```python
from build123d import *

# Parameters (mm, degrees)
F1_DEPTH  = 25
F3_DEPTH  = 75
F5_DEPTH  = 10
F7_R      = 13.8307060356
F7_R_2    = 7.44
F8_DEPTH  = 10
F9_DEPTH  = 35.001
F11_DEPTH = 20
F13_R     = 35.5
F14_DEPTH = 130
F15_R     = 20.5
F16_DEPTH = 223.001
F18_R     = 35.5
F19_DEPTH = 130
F20_R     = 20.5
F21_DEPTH = 210.001
F22_SIZE  = 2


with BuildPart() as f1:
    # F0 (on Top) → F1 (new body)
    with BuildSketch(Plane.XY):
        with BuildLine():
            Line((-190, 0), (-10, 0))
            ThreePointArc((-10, 0), (-2.9289321881, 2.9289321881), (0, 10))
            Line((0, 10), (0, 203))
            ThreePointArc((0, 203), (-2.9289321881, 210.0710678119), (-10, 213))
            Line((-10, 213), (-190, 213))
            ThreePointArc((-190, 213), (-197.0710678119, 210.0710678119), (-200, 203))
            Line((-200, 203), (-200, 10))
            ThreePointArc((-200, 10), (-197.0710678119, 2.9289321881), (-190, 0))
        make_face()
    extrude(amount=F1_DEPTH)

    # F2 (on face) → F3 (join)
    with BuildSketch(Plane.XY.offset(25)):
        with BuildLine():
            Line((0, 155.0000011921), (0, 170))
            Line((0, 170), (-80, 170))
            ThreePointArc((-80, 170), (-106.3603896932, 106.3603896932), (-170, 80))
            Line((-170, 80), (-170, 0))
            Line((-170, 0), (-155, 0))
            Line((-155, 0), (-155, 66.0769515459))
            ThreePointArc((-155, 66.0769515459), (-95.7537875496, 95.7537884012), (-66.0769513738, 155.0000011921))
            Line((-66.0769513738, 155.0000011921), (0, 155.0000011921))
        make_face()
    extrude(amount=F3_DEPTH)

    # F4 (on face) → F5 (join)
    with BuildSketch(Plane.XY.offset(25)):
        with BuildLine():
            Line((0, 60), (-45, 60))
            ThreePointArc((-45, 60), (-55.6066017178, 55.6066017178), (-60, 45))
            Line((-60, 45), (-60, 0))
            Line((-60, 0), (-10, 0))
            ThreePointArc((-10, 0), (-2.9289321881, 2.9289321881), (0, 10))
            Line((0, 10), (0, 60))
        make_face()
    extrude(amount=F5_DEPTH)

    # F7 (on face) → F8 (cut)
    with BuildSketch(Plane.XY.offset(35)):
        with Locations((-30, 30)):
            Circle(F7_R)
        with Locations((-30, 30)):
            Circle(F7_R_2, mode=Mode.SUBTRACT)
    extrude(amount=-F8_DEPTH, mode=Mode.SUBTRACT)

    # F7 (on face) → F9 (cut, through all)
    with BuildSketch(Plane.XY.offset(35)):
        with Locations((-30, 30)):
            Circle(F7_R_2)
    extrude(amount=-F9_DEPTH, mode=Mode.SUBTRACT)

    # F10 (on face) → F11 (cut)
    with BuildSketch(Plane.XY.offset(25)):
        with BuildLine():
            ThreePointArc((-78, 9), (-71.6360389693, 11.6360389693), (-69, 18))
            Line((-69, 18), (-69, 45))
            ThreePointArc((-69, 45), (-61.9705627485, 61.9705627485), (-45, 69))
            Line((-45, 69), (-18, 69))
            ThreePointArc((-18, 69), (-11.6360389693, 71.6360389693), (-9, 78))
            Line((-9, 78), (-9, 137.0000011921))
            ThreePointArc((-9, 137.0000011921), (-11.6360389693, 143.3639622228), (-18, 146.0000011921))
            Line((-18, 146.0000011921), (-51.5094937192, 146.0000011921))
            ThreePointArc((-51.5094937192, 146.0000011921), (-56.9532191654, 144.1669986991), (-60.1795307641, 139.4146352512))
            ThreePointArc((-60.1795307641, 139.4146352512), (-89.3898265392, 89.3898273502), (-139.4146341463, 60.1795310719))
            ThreePointArc((-139.4146341463, 60.1795310719), (-144.1669975344, 56.9532194614), (-146, 51.5094940512))
            Line((-146, 51.5094940512), (-146, 18))
            ThreePointArc((-146, 18), (-143.3639610307, 11.6360389693), (-137, 9))
            Line((-137, 9), (-78, 9))
        make_face()
    extrude(amount=-F11_DEPTH, mode=Mode.SUBTRACT)

    # F13 (on offset) → F14 (join)
    with BuildSketch(Plane.XZ.offset(10)):
        with Locations((-162.5, 100)):
            Circle(F13_R)
    extrude(amount=-F14_DEPTH)

    # F15 (on face) → F16 (cut, through all)
    with BuildSketch(Plane.XZ.offset(10)):
        with Locations((-162.5, 100)):
            Circle(F15_R)
    extrude(amount=-F16_DEPTH, mode=Mode.SUBTRACT)

    # F18 (on offset) → F19 (join)
    with BuildSketch(Plane.YZ.offset(10)):
        with Locations((162.5, 100)):
            Circle(F18_R)
    extrude(amount=-F19_DEPTH)

    # F20 (on face) → F21 (cut, through all)
    with BuildSketch(Plane.YZ.offset(10)):
        with Locations((162.5, 100)):
            Circle(F20_R)
    extrude(amount=-F21_DEPTH, mode=Mode.SUBTRACT)

    # F22
    f22_edges = [f1.edges().sort_by_distance(p)[0] for p in [
        (10, 142, 100),
        (-183, -10, 100),
        (-120, 142, 100),
        (-183, 120, 100),
    ]]
    chamfer(f22_edges, length=F22_SIZE)


solid = f1.part
```
Work out the finished part from the listing and answer in its coordinate system (mm). A direction names the side the tool comes from. Coordinates: 2 decimals unless noted, no trailing zeros. Order: outer loops, then holes, each group sorted by start corner. A loop starts at its lowest first (then second) coordinate and runs counter-clockwise, first axis right, second up. Notation, with made-up numbers: (66, 52) - (89, 52) arc R18 cw to (89, 82) - close; hole circle Ø2 at (75.25, 54). An arc over 180 degrees is marked (long way). Answer as a JSON object with one key per item and string values.
1. Consider line 1 (Z direction, x = -81.5, y = 162); line 2 (Z direction, x = -52, y = 162.5); line 3 (Z direction, x = -149, y = 60). Determine where each line is inside the solid, lowest interval first.
Output values:
{"line 1": "z = 0 to 25, 64.5 to 79.51, 120.49 to 135.5", "line 2": "z = 0 to 79.5, 120.5 to 135.5", "line 3": "z = 0 to 25, 67.17 to 84.57, 115.43 to 132.83"}
2. Find section C-C on z = 11.5. Determine the outline of the cut face in (x, y).
Output values:
{"outline": "(-200, 10) arc R10 ccw to (-190, 0) - (-10, 0) arc R10 ccw to (0, 10) - (0, 203) arc R10 ccw to (-10, 213) - (-190, 213) arc R10 ccw to (-200, 203) - close; hole (-146, 18) arc R9 ccw to (-137, 9) - (-78, 9) arc R9 ccw to (-69, 18) - (-69, 45) arc R24 cw to (-45, 69) - (-18, 69) arc R9 ccw to (-9, 78) - (-9, 137) arc R9 ccw to (-18, 146) - (-51.51, 146) arc R9 ccw to (-60.18, 139.41) arc R114 cw to (-139.41, 60.18) arc R9 ccw to (-146, 51.51) - close; hole circle Ø14.88 at (-30, 30)"}
3. Each of these flat-tipped pins is pushed along its axis until it touches: P1, Ø10, axis at y = 36, z = 17.5, coming from the +X side; P2, Ø4, axis at x = -25.5, y = 190.5, coming from the +Z side; P3, Ø8, axis at x = -50, y = 109, coming from the +Z side. Where does it stop, or does it pass through?
Output values:
{"P1": "stops at x = 0", "P2": "stops at z = 124.17", "P3": "stops at z = 5"}
4. A tool of negligible diameter and unlimited length cuts with its end or side. For faces 4 (the face through (-39, 170, 45)), 5 (the face through (-155, 33, 45)), 6 (the face through (-22, 60, 30)), from which of +Z, -Z, +X, -X, +Y, -Y can it reach the whole face along a straight path? Write none if from no direction.
Output values:
{"face 4": "+X, -X, +Y", "face 5": "-Y", "face 6": "+Z, +X"}
5. Find section D-D on y = 162.5. Determine the outline of the cut face in (x, z).
Output values:
{"outline": "(-200, 0) - (0, 0) - (0, 64.5) - (10, 64.5) - (10, 77.5) - (8, 79.5) - (-118, 79.5) - (-120, 77.5) - (-120, 64.5) - (-80.31, 64.5) - (-80.31, 25) - (-200, 25) - close; (-120, 122.5) - (-118, 120.5) - (8, 120.5) - (10, 122.5) - (10, 135.5) - (-120, 135.5) - close"}
6. Find section B-B on z = 32. Determine the outline of the cut face in (x, y).
Output values:
{"outline": "(-170, 0) - (-155, 0) - (-155, 66.08) arc R105 ccw to (-66.08, 155) - (0, 155) - (0, 170) - (-80, 170) arc R90 cw to (-170, 80) - close; (-60, 0) - (-10, 0) arc R10 ccw to (0, 10) - (0, 60) - (-45, 60) arc R15 ccw to (-60, 45) - close; hole circle Ø27.66 at (-30, 30)"}
7. Find section A-A on x = -30. Determine the outline of the cut face in (y, z).
Output values:
{"outline": "(0, 0) - (22.56, 0) - (22.56, 25) - (16.17, 25) - (16.17, 35) - (0, 35) - close; (37.44, 0) - (213, 0) - (213, 25) - (170, 25) - (170, 65.3) arc R35.5 ccw (long way) to (155, 65.3) - (155, 25) - (146, 25) - (146, 5) - (69, 5) - (69, 25) - (60, 25) - (60, 35) - (43.83, 35) - (43.83, 25) - (37.44, 25) - close; hole circle Ø41 at (162.5, 100)"}
8. The mould has two halves that part along Y. Classify faces 1 (the face through (-2.85, 209.99, 12.32)), 2 (the face through (-54.12, 146.23, 87.53)), 3 (the face through (-101, 0, 18)): +Y half, -Y half, draft (parallel to the pull), parting line (faces both ways), or undercut.
Output values:
{"face 1": "+Y half", "face 2": "undercut", "face 3": "-Y half"}
